```python
from build123d import *

# Parameters (mm, degrees)
F0_W     = 145.4039812088
F0_H     = 34.9461883307
F1_DEPTH = 78.74
F5_DEPTH = 25.4


# Not quite as in the source:
# - the program builds the solid bodies; features that only make, move or delete a surface that nothing else refers to are left out


with BuildPart() as f1:
    # F0 (on Top) → F1 (new body)
    with BuildSketch(Plane.XY):
        with Locations((72.7019906044, 72.0167830586)):
            Rectangle(F0_W, F0_H)
    extrude(amount=F1_DEPTH)

    # F4 (on face) → F5 (cut)
    with BuildSketch(Plane.XY.offset(78.74)):
        with BuildLine():
            Line((145.4039812088, 54.5436888933), (145.4039812088, 72.0167830586))
            ThreePointArc((145.4039812088, 72.0167830586), (115.6911009346, 79.8555366854), (97.9683505694, 54.7516439176))
            Line((97.9683505694, 54.7516439176), (145.4039812088, 54.5436888933))
        make_face()
    extrude(amount=-F5_DEPTH, mode=Mode.SUBTRACT)


solid = f1.part
```
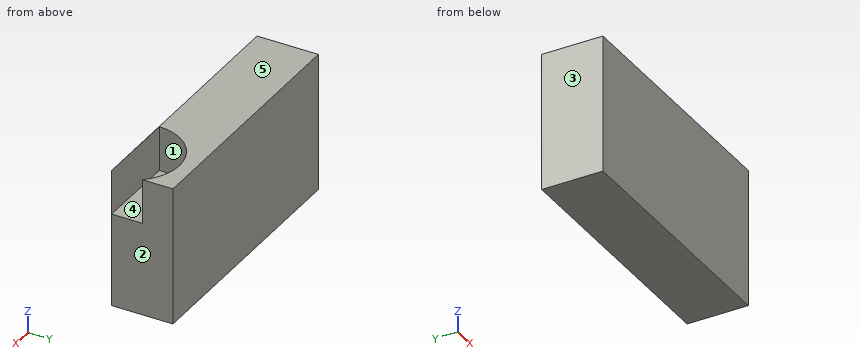
Geometry check sheet. Reference: the model listing, model coordinates, mm. Face numbers are marked on the shaded views. A direction names the side the tool comes from. Give positions to 0.01 mm unless a question says otherwise; leave off trailing zeros. Loops run counter-clockwise (first coordinate to the right, second up) from the corner with the lowest first, then second, coordinate; pieces in that order, holes last. Notation, with made-up numbers: M -40,-14 L -7,-14 A33 cw -7,15 Z; hole C 43,86.25 d10. An arc over 180 degrees is marked long. Answer as CSV lines item,"result".
Item 1: Cross-section at D-D on y = 58.5. Record the cut outline in (x, z).
Values:
outline,"M 0,0 L 145.4,0 L 145.4,53.34 L 98.26,53.34 L 98.26,78.74 L 0,78.74 Z"
Item 2: Release check for a two-part mould opening along X. For the marked faces 3, 4 and 5 record: pulls with the +X half, pulls with the -X half, needs draft (parallel to the pull), parting line crosses it, or undercut.
Values:
face 3,"pulls with the -X half"
face 4,"undercut"
face 5,"needs draft"
Item 3: Material ranges on line 1 (Z direction, x = 102.5, y = 63); line 2 (X direction, y = 74, z = 69); line 3 (X direction, y = 64, z = 55.5), recorded low to high.
Values:
line 1,"z = 0 to 53.34"
line 2,"x = 0 to 106.28, 143.53 to 145.4"
line 3,"x = 0 to 99.68"
Item 4: Cross-section at C-C on z = 70. Record the cut outline in (x, y), and give its area (3 significant figures).
Values:
outline,"M 0,54.54 L 145.4,54.54 L 97.97,54.75 A26.94 cw 145.4,72.02 L 145.4,89.49 L 0,89.49 Z"
area,"4,020 mm²"
Item 5: Cross-section at A-A on x = 125. Record the cut outline in (y, z), and give its area (3 significant figures).
Values:
outline,"M 54.54,0 L 89.49,0 L 89.49,78.74 L 81.48,78.74 L 81.48,53.34 L 54.63,53.34 L 54.63,78.74 L 54.54,78.74 Z"
area,"2,070 mm²"
Item 6: Access from +Z, -Z, +X, -X, +Y, -Y to the whole of each face (thin tool, end or side, straight path). Record for the marked faces 1 and 2.
Values:
face 1,"+Z"
face 2,"+Z, -Z, +X, +Y, -Y"
Item 7: Cross-section at B-B on y = 79. Record the cut outline in (x, z), and give its area (3 significant figures).
Values:
outline,"M 0,0 L 145.4,0 L 145.4,78.74 L 136.19,78.74 L 136.19,53.34 L 113.61,53.34 L 113.61,78.74 L 0,78.74 Z"
area,"10,900 mm²"
